Design review of the part built by this model. Coordinates are the model's own, in mm. A direction names the side the tool comes from. Coordinates: 2 decimals unless noted, no trailing zeros. Write each loop counter-clockwise with the first axis right and the second up, starting at its lowest first coordinate (ties: lowest second). Pieces come first, ordered by that corner, then holes.
Q1. The part is to be moulded in two halves that separate along X. For faces 3 (the flat face through (0, 3.175, -3)), 4 (the cylindrical face through (-1.89, 1.61, -1.45)), 5 (the cylindrical face through (-1.38, 3.53, -6.2)), 6 (the flat face through (1.44, 7.144, 4.15)), say which applies: released by +X, released by -X, zero draft, split by the parting line, or undercut.
Q2. For pin 1 Ø6 at (x, z) = (0, 0) entering from +Y (3 decimals); pin 2 Ø1 at (x, y) = (-1, 2.5) entering from +Z, all flat-tipped, find the tip position at first contact; note any pin that passes through.
Q3. For faces 1 (the cylindrical face through (-0.86, 5.254, -3.874)), 2 (the flat face through (3, 0, -1)), list the 3-axis set-ups (+Z, -Z, +X, -X, +Y, -Y) from which the entire face can be reached by the end or side of a thin tool; tool diameter is ignored.
Q4. Take a section at C-C, the plane y = 1.25. Write out the cut boundary in (x, z).
Q5. For L1, parallel to Z at x = 0, y = 1.45; L2, parallel to Z at x = 0, y = 4.5; L3, parallel to Y at x = 1.5, z = -3.25, list the stretches that pass through material, from the lowest coordinate up.
Q6. Take a section at D-D, the plane y = 5.5. Write out the cut boundary in (x, z), plus the area to 3 significant figures.
Q7. Take a section at B-B, the plane z = 0. Write out the cut boundary in (x, y) (3 decimals), plus the area to 3 significant figures.
Q8. Take a section at A-A, the plane x = 0. Write out the cut boundary in (y, z) (3 decimals).
from build123d import *

# Parameters (mm, degrees)
FILLET1_R     = 0.396875
CHAMFER1_SIZE = 0.254


with BuildPart() as part:
    # Sketch1 → Revolve1 (revolve)
    with BuildSketch(Plane.XY):
        Polygon((2.38125, 0), (2.38125, 3.175), (3.96875, 3.175), (3.96875, 7.14375), (6.35, 7.14375), (6.35, 0), align=None)
    revolve(axis=Axis((0, 0, 0), (0, -1, 0)))

    # Fillet1
    fillet1_edges = [part.edges().sort_by_distance(p)[0] for p in [
        (-3.96875, 3.175, 0),
    ]]
    fillet(fillet1_edges, radius=FILLET1_R)

    # Chamfer1
    chamfer1_edges = [part.edges().sort_by_distance(p)[0] for p in [
        (-6.35, 0, 0),
        (-6.35, 7.14375, 0),
        (-3.96875, 7.14375, 0),
        (-2.38125, 3.175, 0),
        (-2.38125, 0, 0),
    ]]
    chamfer(chamfer1_edges, length=CHAMFER1_SIZE)


solid = part.part
Responses:
1. face 3: undercut
1. face 4: undercut
1. face 5: split by the parting line
1. face 6: zero draft
2. pin 1: stops at y = 3.175
2. pin 2: stops at z = 6.33
3. face 1: +Y
3. face 2: +Z, -Z, +X, -X, -Y
4. outline: circle Ø12.7 at (0, 0); hole circle Ø4.76 at (0, 0)
5. L1: z = -6.35 to -2.38, 2.38 to 6.35
5. L2: z = -6.35 to -3.97, 3.97 to 6.35
5. L3: y = 0 to 3.18
6. outline: circle Ø12.7 at (0, 0); hole circle Ø7.94 at (0, 0)
6. area: 77.2 mm2
7. outline: (-6.35, 0.254) - (-6.096, 0) - (-2.635, 0) - (-2.381, 0.254) - (-2.381, 2.921) - (-2.635, 3.175) - (-3.572, 3.175) arc R0.397 cw to (-3.969, 3.572) - (-3.969, 6.89) - (-4.223, 7.144) - (-6.096, 7.144) - (-6.35, 6.89) - close; (2.381, 0.254) - (2.635, 0) - (6.096, 0) - (6.35, 0.254) - (6.35, 6.89) - (6.096, 7.144) - (4.223, 7.144) - (3.969, 6.89) - (3.969, 3.572) arc R0.397 cw to (3.572, 3.175) - (2.635, 3.175) - (2.381, 2.921) - close
7. area: 43.8 mm2
8. outline: (0, -6.096) - (0.254, -6.35) - (6.89, -6.35) - (7.144, -6.096) - (7.144, -4.223) - (6.89, -3.969) - (3.572, -3.969) arc R0.397 cw to (3.175, -3.572) - (3.175, -2.635) - (2.921, -2.381) - (0.254, -2.381) - (0, -2.635) - close; (0, 2.635) - (0.254, 2.381) - (2.921, 2.381) - (3.175, 2.635) - (3.175, 3.572) arc R0.397 cw to (3.572, 3.969) - (6.89, 3.969) - (7.144, 4.223) - (7.144, 6.096) - (6.89, 6.35) - (0.254, 6.35) - (0, 6.096) - close
